Answer from the drawing. Dimensions are ordinates in mm from the lowest x, y and z of the part. A direction names the side the tool comes from. Coordinates: 2 decimals unless noted, no trailing zeros. Write each loop counter-clockwise with the first axis right and the second up, starting at its lowest first coordinate (ties: lowest second). Pieces come first, ordered by that corner, then holes. Notation, with made-up numbers: M 63,37.5 L 101,37.5 A35 ccw 101,73.5 Z; hole C 50.5,-5.5 d3. An arc over 180 degrees is marked long. Put each result on its own line as item: value. Start each with the question number.
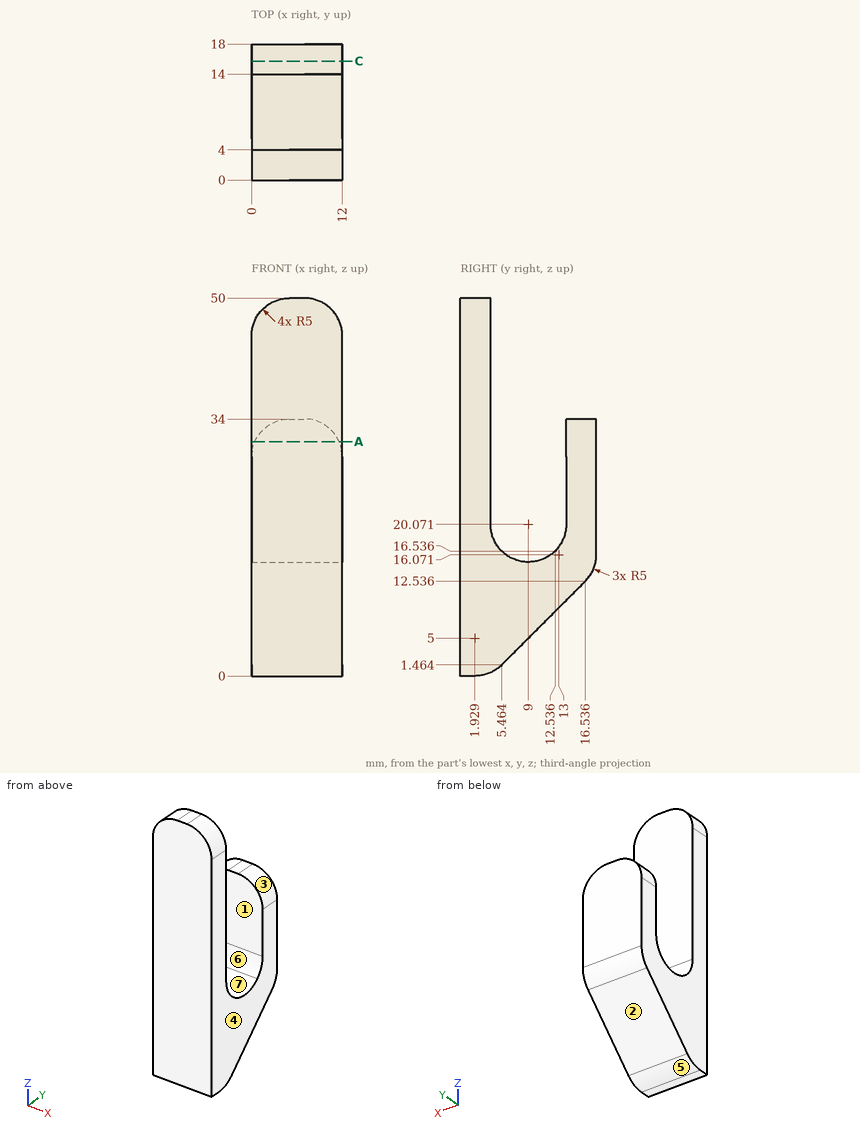
1) A cutting plane is placed at C-C on y = 15.75. Write down the section's boundary in (x, z), then the cut area to 3 significant figures.
2) Given pin 1 Ø2 at (x, y) = (6, 16) entering from +Z; pin 2 Ø3 at (x, y) = (2, 4.5) entering from +Z, each flat-ended and moving along its own axis, determine where each tip first touches the part or whether it passes through.
3) For the marked faces 1, 2 and 3, determine the directions among +Z, -Z, +X, -X, +Y, -Y from which every point of the face is accessible in a straight line to the end or side of a thin tool.
4) Straight lines are drawn through the part: probe 1 along Y at (x, z) = (10, 26); probe 2 along Y at (x, z) = (1, 42); probe 3 along Z at (x, y) = (6.25, 16). For each, find the intervals that lie inside material, in ascending order.
5) A cutting plane is placed at A-A on z = 31. Write down the section's boundary in (x, y).
6) Determine the mould class of the marked faces 4, 5, 6 and 7 for opening direction Y: +Y half, -Y half, draft (parallel to the pull), parting line (faces both ways), or undercut.
Answers follow:
1. outline: M 0,11.75 L 12,11.75 L 12,29 A5 ccw 7,34 L 5,34 A5 ccw 0,29 Z
1. area: 256 mm²
2. pin 1: stops at z = 34
2. pin 2: stops at z = 49.74
3. face 1: +Z, +X, -X
3. face 2: -Z, +X, -X, +Y
3. face 3: +Z, +X, +Y
4. probe 1: y = 0 to 4, 14 to 18
4. probe 2: y = 0 to 4
4. probe 3: z = 12 to 34
5. outline: M 0,0 L 12,0 L 12,4 L 0,4 Z; M 0.42,14 L 11.58,14 L 11.58,18 L 0.42,18 Z
6. face 4: draft
6. face 5: +Y half
6. face 6: undercut
6. face 7: undercut
